from build123d import *

# Parameters (mm, degrees)
SKETCH_2_R      = 2.75
EXTRUDE_1_DEPTH = 1.5
SKETCH_3_R      = 21
EXTRUDE_2_DEPTH = 17
FILLET_4_R      = 3
SKETCH_6_R      = 14.75
EXTRUDE_3_DEPTH = 7.5
FILLET_3_R      = 2
FILLET_7_R      = 25
FILLET_8_R      = 5


with BuildPart() as part:
    # ｽｹｯﾁ2 → ﾎﾞｽ - 押し出し1 (new body)
    with BuildSketch(Plane.XY):
        Polygon((0, -35), (-36, 0), (0, 35), (36, 0), align=None)
        with Locations((-28, 0)):
            Circle(SKETCH_2_R, mode=Mode.SUBTRACT)
        with Locations((28, 0)):
            Circle(SKETCH_2_R, mode=Mode.SUBTRACT)
    extrude(amount=EXTRUDE_1_DEPTH)

    # ｽｹｯﾁ3 → ﾎﾞｽ - 押し出し2 (add)
    with BuildSketch(Plane.XY.offset(1.5)):
        Circle(SKETCH_3_R)
    extrude(amount=-EXTRUDE_2_DEPTH)

    # ﾌｨﾚｯﾄ4
    fillet_4_edges = [part.edges().sort_by_distance(p)[0] for p in [
        (-21, 0, -15.5),
    ]]
    fillet(fillet_4_edges, radius=FILLET_4_R)

    # ｽｹｯﾁ5 → 回転1 (revolve)
    with BuildSketch(Plane(origin=(0, 0, -16.8), x_dir=(-1, 0, 0), z_dir=(0, 0, -1))):
        with BuildLine():
            Line((0, 12.7), (0, -12.7))
            ThreePointArc((0, -12.7), (-12.7, 0), (0, 12.7))
        make_face()
    revolve(axis=Axis((0, -12.7, -16.8), (0, 1, 0)))

    # ｽｹｯﾁ6 → ﾎﾞｽ - 押し出し3 (add)
    with BuildSketch(Plane(origin=(0, 0, -15.5), x_dir=(-1, 0, 0), z_dir=(0, 0, -1))):
        with Locations(Location((0, 0, 0), (0, 0, 180))):
            Circle(SKETCH_6_R)
    extrude(amount=EXTRUDE_3_DEPTH)

    # ﾌｨﾚｯﾄ3
    fillet_3_edges = [part.edges().sort_by_distance(p)[0] for p in [
        (-14.75, 0, -23),
    ]]
    fillet(fillet_3_edges, radius=FILLET_3_R)

    # ﾌｨﾚｯﾄ7
    fillet_7_edges = [part.edges().sort_by_distance(p)[0] for p in [
        (0, 35, 0.75),
        (0, -35, 0.75),
    ]]
    fillet(fillet_7_edges, radius=FILLET_7_R)

    # ﾌｨﾚｯﾄ8
    fillet_8_edges = [part.edges().sort_by_distance(p)[0] for p in [
        (36, 0, 0.75),
        (-36, 0, 0.75),
    ]]
    fillet(fillet_8_edges, radius=FILLET_8_R)


solid = part.part
Model file for the job. Use its own axes, mm. A direction names the side the tool comes from. Give positions to 0.01 mm unless a question says otherwise; leave off trailing zeros. Order: outer loops, then holes, each group sorted by start corner. A loop starts at its lowest first (then second) coordinate and runs counter-clockwise, first axis right, second up. Notation, with made-up numbers: (3.25, 69.25) - (48.25, 69.25) arc R12 ccw to (48.25, 77.25) - close; hole circle Ø6 at (10, -35.75). An arc over 180 degrees is marked (long way). One line per item, written item: value.
Item 1: Wall check: line 1 (Y direction, x = 28, z = 0.7); line 2 (Z direction, x = 10.5, y = -13); line 3 (Z direction, x = 23, y = 3). Give the ranges that are in metal, low to high.
Response values:
line 1: -7.78 to -2.75, 2.75 to 7.78
line 2: -15.5 to 1.5
line 3: 0 to 1.5
Item 2: Pin check, flat tips, straight feed: pin 1 Ø15 at (x, y) = (-1.5, 4.5) entering from -Z; pin 2 Ø8 at (y, z) = (-6, -15) entering from -X; pin 3 Ø8 at (y, z) = (-9.5, -8.5) entering from +X; pin 4 Ø9 at (x, y) = (28, 0) entering from +Z. Stop position of each tip, or through.
Response values:
pin 1: z = -29.5
pin 2: x = -20.82
pin 3: x = 20.27
pin 4: z = 1.5
Item 3: Slice it at D-D (z = -5). List the corners of the cut face in (x, y), then the cut area to 3 significant figures.
Response values:
outline: circle Ø42 at (0, 0)
area: 1,390 mm2
Item 4: Slice it at A-A (y = 0). List the corners of the cut face in (x, z).
Response values:
outline: (-33.83, 0) - (-30.75, 0) - (-30.75, 1.5) - (-33.83, 1.5) - close; (-25.25, 0) - (-21, 0) - (-21, -12.5) arc R3 ccw to (-18, -15.5) - (-14.75, -15.5) - (-14.75, -21) arc R2 ccw to (-12.75, -23) - (-11.08, -23) arc R12.7 ccw to (11.08, -23) - (12.75, -23) arc R2 ccw to (14.75, -21) - (14.75, -15.5) - (18, -15.5) arc R3 ccw to (21, -12.5) - (21, 0) - (25.25, 0) - (25.25, 1.5) - (-25.25, 1.5) - close; (30.75, 0) - (33.83, 0) - (33.83, 1.5) - (30.75, 1.5) - close
Item 5: Tool access for faces 1 (the cylindrical face through (14.07, -4.43, -18.21)), 2 (the flat face through (0, 0, 1.5)): list every direction of +Z, -Z, +X, -X, +Y, -Y with a clear straight run to the whole face (end or side of a thin tool).
Response values:
face 1: -Z
face 2: +Z, +X, -X, +Y, -Y
Item 6: Slice it at B-B (x = -27.5). List the corners of the cut face in (y, z), then the cut area to 3 significant figures.
Response values:
outline: (-8.26, 0) - (-2.7, 0) - (-2.7, 1.5) - (-8.26, 1.5) - close; (2.7, 0) - (8.26, 0) - (8.26, 1.5) - (2.7, 1.5) - close
area: 16.7 mm2
Item 7: Slice it at C-C (x = 0). List the corners of the cut face in (y, z).
Response values:
outline: (-25.13, 0) - (-21, 0) - (-21, -12.5) arc R3 ccw to (-18, -15.5) - (-14.75, -15.5) - (-14.75, -21) arc R2 ccw to (-12.75, -23) - (-11.08, -23) arc R12.7 ccw to (11.08, -23) - (12.75, -23) arc R2 ccw to (14.75, -21) - (14.75, -15.5) - (18, -15.5) arc R3 ccw to (21, -12.5) - (21, 0) - (25.13, 0) - (25.13, 1.5) - (-25.13, 1.5) - close
